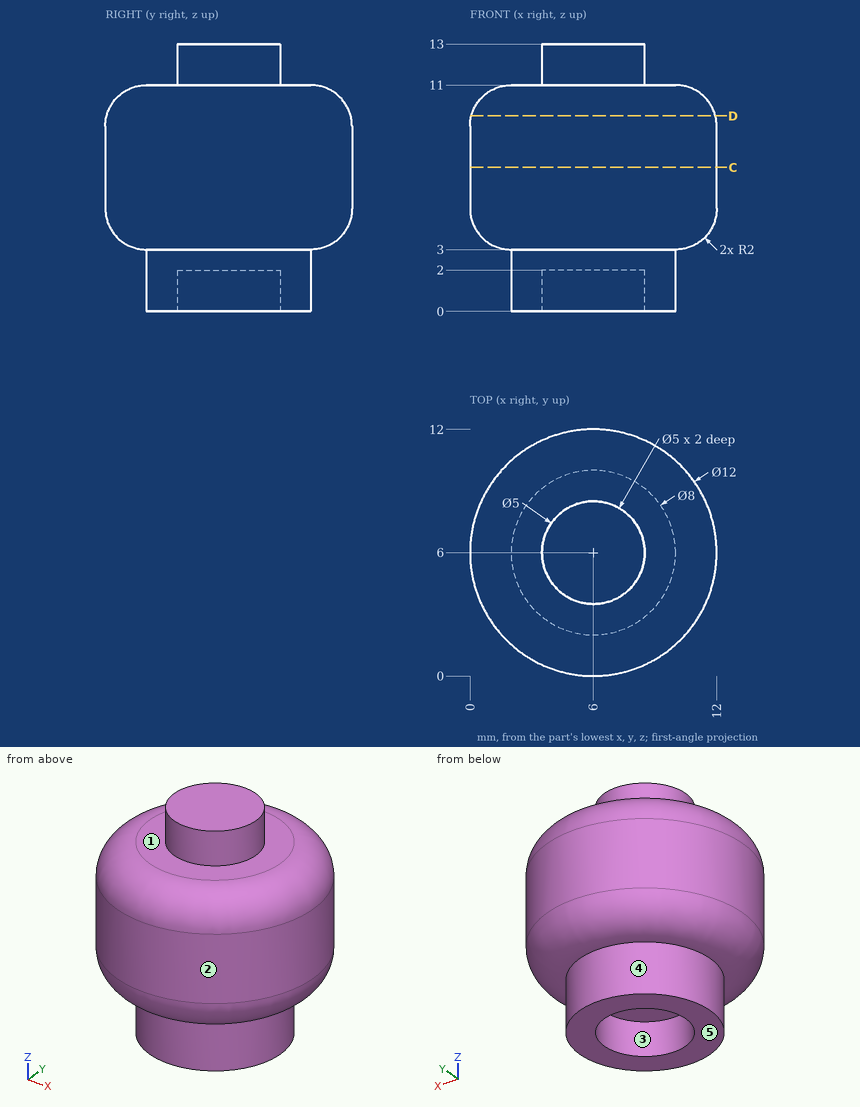
Drawing for the job (mm, zero at the part's lowest x, y, z). A direction names the side the tool comes from. Round coordinates to 2 decimals unless told otherwise and drop trailing zeros. Loops run counter-clockwise (first coordinate to the right, second up) from the corner with the lowest first, then second, coordinate; pieces in that order, holes last. Notation, with made-up numbers: (6.25, -1.5) - (24.25, -1.5) arc R33 ccw to (24.25, 33.5) - close; hole circle Ø3 at (24, 19.25). An arc over 180 degrees is marked (long way). Return JSON: item names as keys, results as strings. Group by question number.
Q1. Tool access for the marked faces 1 and 2: list every direction of +Z, -Z, +X, -X, +Y, -Y with a clear straight run to the whole face (end or side of a thin tool).
Q2. Band-saw the part on C-C on z = 7. Give the cut face in (x, y), plus the area to 3 significant figures.
Q3. Drill centre lines: line 1 along Y through (x, z) = (6, 0.5); line 2 along Z through (x, y) = (5.5, 5); line 3 along Z through (x, y) = (8.5, 4.25). Where is each one in solid material? Low to high. Write a range as [from, to].
Q4. Flat gauge pins, fed straight in: pin 1 Ø3 at (x, y) = (6, 6) entering from -Z; pin 2 Ø1.5 at (x, z) = (5.5, 2.5) entering from +Y (3 decimals); pin 3 Ø1 at (x, z) = (2.5, 3.5) entering from +Y. Where does each tip first touch, or does it go through?
Q5. Two-plate mould, pull along Y, no slides. Class the marked faces 3, 4 and 5: +Y half, -Y half, draft (parallel to the pull), parting line (faces both ways), or undercut.
Q6. Band-saw the part on D-D on z = 9.5. Give the cut face in (x, y), plus the area to 3 significant figures.
Solutions:
{
 "1": {"face 1": "+Z", "face 2": "+Z, -Z"},
 "2": {"outline": "circle Ø12 at (6, 6)", "area": "113 mm^2"},
 "3": {"line 1": "y = [2, 3.5], [8.5, 10]", "line 2": "z = [2, 13]", "line 3": "z = [0, 11]"},
 "4": {"pin 1": "stops at z = 2", "pin 2": "stops at y = 10.945", "pin 3": "stops at y = 10.68"},
 "5": {"face 3": "undercut", "face 4": "parting line", "face 5": "draft"},
 "6": {"outline": "circle Ø11.87 at (6, 6)", "area": "111 mm^2"}
}
